For this review, take the finished solid that the model builds, in its own axes (mm). A direction names the side the tool comes from. Coordinates: 2 decimals unless noted, no trailing zeros. Loops run counter-clockwise (first coordinate to the right, second up) from the corner with the lowest first, then second, coordinate; pieces in that order, holes last. Notation, with made-up numbers: (-28, 61) -> (-23, 61) arc R28 cw to (-23, 80) -> close; hole circle Ø7 at (47.25, 51). An arc over 180 degrees is marked (long way). One line per item, written item: value.
from build123d import *

# Parameters (mm, degrees)
SKETCH2_R           = 1.5
BOSS_EXTRUDE1_DEPTH = 8.7
SKETCH3_R           = 4
SKETCH3_R_2         = 2.55
BOSS_EXTRUDE2_DEPTH = 2.5
BOSS_EXTRUDE3_START = -11.2
SKETCH3_3_R         = 4
SKETCH3_3_R_2       = 2.55
BOSS_EXTRUDE3_DEPTH = 2.5
CUT_EXTRUDE1_START  = -0.5
SKETCH2_3_R         = 5
SKETCH2_3_R_2       = 2.55
CUT_EXTRUDE1_DEPTH  = 9.7
BOSS_EXTRUDE4_START = -2.5
SKETCH2_4_R         = 2.55
BOSS_EXTRUDE4_DEPTH = 0.5
FILLET1_R           = 10
FILLET2_R           = 0.5
FILLET3_R           = 1


with BuildPart() as part:
    # Sketch2 → Boss-Extrude1 (new body)
    with BuildSketch(Plane(origin=(0, 0, 0), x_dir=(1, 0, 0), z_dir=(0, 1, 0))):
        with BuildLine():
            Line((3.9, 3.65), (-3.9, 3.65))
            Line((-3.9, 3.65), (-3.9, -3.65))
            Line((-3.9, -3.65), (-5, -3.65))
            Line((-5, -3.65), (-5, -6.15))
            Line((-5, -6.15), (-3.9, -6.15))
            Line((-3.9, -6.15), (-3.9, -21.871102431))
            ThreePointArc((-3.9, -21.871102431), (0, -20), (3.9, -21.871102431))
            Line((3.9, -21.871102431), (3.9, -6.15))
            Line((3.9, -6.15), (5, -6.15))
            Line((5, -6.15), (5, -3.65))
            Line((5, -3.65), (3.9, -3.65))
            Line((3.9, -3.65), (3.9, 3.65))
        make_face()
        with Locations(Location((0, 0.2, 0), (0, 0, 270))):
            Circle(SKETCH2_R, mode=Mode.SUBTRACT)
    extrude(amount=BOSS_EXTRUDE1_DEPTH)

    # Sketch3 → Boss-Extrude2 (add)
    # profile 1 of 4: a face of its own
    with BuildSketch(Plane(origin=(0, 8.7, 0), x_dir=(1, 0, 0), z_dir=(0, 1, 0))):
        Polygon((-5, -3.65), (-5, -6.15), (-3.9, -6.15), (3.9, -6.15), (5, -6.15), (5, -3.65), (3.9, -3.65), (-3.9, -3.65), align=None)
    # profile 2 of 4: a face of its own
    with BuildSketch(Plane(origin=(0, 8.7, 0), x_dir=(1, 0, 0), z_dir=(0, 1, 0))):
        with BuildLine():
            Line((3.9, -6.15), (-3.9, -6.15))
            Line((-3.9, -6.15), (-3.9, -21.871102431))
            ThreePointArc((-3.9, -21.871102431), (0, -20), (3.9, -21.871102431))
            Line((3.9, -21.871102431), (3.9, -6.15))
        make_face()
    # profile 3 of 4: a face of its own
    with BuildSketch(Plane(origin=(0, 8.7, 0), x_dir=(1, 0, 0), z_dir=(0, 1, 0))):
        with Locations((0, -25)):
            Circle(SKETCH3_R)
        with Locations(Location((0, -25, 0), (0, 0, 270))):
            Circle(SKETCH3_R_2, mode=Mode.SUBTRACT)
    # profile 4 of 4: a face of its own
    with BuildSketch(Plane(origin=(0, 8.7, 0), x_dir=(1, 0, 0), z_dir=(0, 1, 0))):
        with BuildLine():
            ThreePointArc((3.9, -21.871102431), (0, -20), (-3.9, -21.871102431))
            Line((-3.9, -21.871102431), (-3.9, -24.111180558))
            ThreePointArc((-3.9, -24.111180558), (0, -21), (3.9, -24.111180558))
            Line((3.9, -24.111180558), (3.9, -21.871102431))
        make_face()
    extrude(amount=BOSS_EXTRUDE2_DEPTH)

    # Sketch3<3> → Boss-Extrude3 (add)
    # profile 1 of 4: a face of its own
    with BuildSketch(Plane(origin=(0, 8.7, 0), x_dir=(1, 0, 0), z_dir=(0, 1, 0)).offset(BOSS_EXTRUDE3_START)):
        with Locations((0, -25)):
            Circle(SKETCH3_3_R)
        with Locations(Location((0, -25, 0), (0, 0, 270))):
            Circle(SKETCH3_3_R_2, mode=Mode.SUBTRACT)
    # profile 2 of 4: a face of its own
    with BuildSketch(Plane(origin=(0, 8.7, 0), x_dir=(1, 0, 0), z_dir=(0, 1, 0)).offset(BOSS_EXTRUDE3_START)):
        with BuildLine():
            ThreePointArc((3.9, -21.871102431), (0, -20), (-3.9, -21.871102431))
            Line((-3.9, -21.871102431), (-3.9, -24.111180558))
            ThreePointArc((-3.9, -24.111180558), (0, -21), (3.9, -24.111180558))
            Line((3.9, -24.111180558), (3.9, -21.871102431))
        make_face()
    # profile 3 of 4: a face of its own
    with BuildSketch(Plane(origin=(0, 8.7, 0), x_dir=(1, 0, 0), z_dir=(0, 1, 0)).offset(BOSS_EXTRUDE3_START)):
        with BuildLine():
            Line((3.9, -6.15), (-3.9, -6.15))
            Line((-3.9, -6.15), (-3.9, -21.871102431))
            ThreePointArc((-3.9, -21.871102431), (0, -20), (3.9, -21.871102431))
            Line((3.9, -21.871102431), (3.9, -6.15))
        make_face()
    # profile 4 of 4: a face of its own
    with BuildSketch(Plane(origin=(0, 8.7, 0), x_dir=(1, 0, 0), z_dir=(0, 1, 0)).offset(BOSS_EXTRUDE3_START)):
        Polygon((-5, -3.65), (-5, -6.15), (-3.9, -6.15), (3.9, -6.15), (5, -6.15), (5, -3.65), (3.9, -3.65), (-3.9, -3.65), align=None)
    extrude(amount=BOSS_EXTRUDE3_DEPTH)

    # Sketch2<3> → Cut-Extrude1 (cut)
    with BuildSketch(Plane(origin=(0, 0, 0), x_dir=(1, 0, 0), z_dir=(0, 1, 0)).offset(CUT_EXTRUDE1_START)):
        with Locations((0, -25)):
            Circle(SKETCH2_3_R)
        with Locations(Location((0, -25, 0), (0, 0, 270))):
            Circle(SKETCH2_3_R_2, mode=Mode.SUBTRACT)
    extrude(amount=CUT_EXTRUDE1_DEPTH, mode=Mode.SUBTRACT)

    # Sketch2<4> → Boss-Extrude4 (add)
    with BuildSketch(Plane(origin=(0, 0, 0), x_dir=(1, 0, 0), z_dir=(0, 1, 0)).offset(BOSS_EXTRUDE4_START)):
        with Locations(Location((0, -25, 0), (0, 0, 270))):
            Circle(SKETCH2_4_R)
    extrude(amount=BOSS_EXTRUDE4_DEPTH)

    # Fillet1
    # the kernel refuses this fillet: 10 mm, written as the material it adds along each edge
    with BuildSketch(Plane(origin=(-3.9, -2.5, 6.15), x_dir=(-1, 0, 0), z_dir=(0, 1, 0)), Plane(origin=(3.9, 11.2, 6.15), x_dir=(1, 0, 0), z_dir=(0, -1, 0))) as fillet1_piece_1:
        with BuildLine():
            CenterArc((10, 4.559605246), FILLET1_R, 180, 27.126753117)
            Line((0, 4.559605246), (-0.2, 4.559605246))
            Line((-0.2, 4.559605246), (-0.2, 0))
            Line((-0.2, 0), (0, -0.2))
            ThreePointArc((0, -0.2), (0.55, -0.2), (0.922, -0.091192105))
            Line((0.922, -0.091192105), (1.1, 0))
        make_face()
    extrude(amount=13.7)

    # Fillet2
    fillet2_edges = [part.edges().sort_by_distance(p)[0] for p in [
        (3.9, 4.35, 21.871102431),
        (-3.9, 4.35, 21.871102431),
    ]]
    fillet(fillet2_edges, radius=FILLET2_R)

    # Fillet3
    fillet3_edges = [part.edges().sort_by_distance(p)[0] for p in [
        (5, 4.35, 3.65),
        (-5, 4.35, 3.65),
        (-3.9, 4.35, -3.65),
        (3.9, 4.35, -3.65),
    ]]
    fillet(fillet3_edges, radius=FILLET3_R)


solid = part.part
1. Insertion check: pin 1 Ø6 at (y, z) = (7.5, 10.5) entering from +X; pin 2 Ø4 at (x, z) = (-0.5, 26) entering from +Y; pin 3 Ø5 at (y, z) = (6.5, 0.5) entering from +X; pin 4 Ø2 at (x, z) = (1.5, 0) entering from +Y. Each pin has a flat end and moves straight along its axis. Give the tip position at first contact, or say it passes through.
Return value:
pin 1: stops at x = 4.43
pin 2: stops at y = 11.2
pin 3: stops at x = 3.9
pin 4: stops at y = 8.7
2. Take a section at B-B, the plane x = 0. Give the boundary of the cut face in (y, z).
Return value:
outline: (-2.5, 3.65) -> (0, 3.65) -> (0, 1.3) -> (8.7, 1.3) -> (8.7, 3.65) -> (11.2, 3.65) -> (11.2, 22.45) -> (9.2, 22.45) -> (9.2, 20) -> (-0.5, 20) -> (-0.5, 22.45) -> (-2, 22.45) -> (-2, 27.55) -> (-0.5, 27.55) -> (-0.5, 29) -> (-2.5, 29) -> close; (0, -3.65) -> (8.7, -3.65) -> (8.7, -1.7) -> (0, -1.7) -> close; (9.2, 27.55) -> (11.2, 27.55) -> (11.2, 29) -> (9.2, 29) -> close
3. Take a section at D-D, the plane y = 2. Give the boundary of the cut face in (x, z).
Return value:
outline: (-5, 4.65) arc R1 ccw to (-4, 3.65) -> (-3.9, 3.65) -> (-3.9, -2.65) arc R1 ccw to (-2.9, -3.65) -> (2.9, -3.65) arc R1 ccw to (3.9, -2.65) -> (3.9, 3.65) -> (4, 3.65) arc R1 ccw to (5, 4.65) -> (5, 6.15) arc R10 cw to (3.9, 10.71) -> (3.9, 20.68) arc R0.5 ccw to (3.09, 21.07) arc R5 cw to (-3.09, 21.07) arc R0.5 ccw to (-3.9, 20.68) -> (-3.9, 10.71) arc R10 cw to (-5, 6.15) -> close; hole circle Ø3 at (0, -0.2)
4. Take a section at C-C, the plane z = -0.2. Give the boundary of the cut face in (x, y), and give its area (3 significant figures).
Return value:
outline: (-3.9, 0) -> (-1.5, 0) -> (-1.5, 8.7) -> (-3.9, 8.7) -> close; (1.5, 0) -> (3.9, 0) -> (3.9, 8.7) -> (1.5, 8.7) -> close
area: 41.8 mm2
5. For faces 4 (the cylindrical face through (3.61, 4.42, 21.13)), 5 (the flat face through (5, 4, 5)), 6 (the flat face through (-3.9, 4, 16)), 7 (the flat face through (0, -2, 25)), 8 (the flat face through (3.9, 4, 1)), list the 3-axis set-ups (+Z, -Z, +X, -X, +Y, -Y) from which the entire face can be reached by the end or side of a thin tool; tool diameter is ignored.
Return value:
face 4: +Z
face 5: +Z, -Z, +X, +Y, -Y
face 6: -X, +Y, -Y
face 7: +Y
face 8: -Z, +X, +Y, -Y
6. The part is to be moulded in two halves that separate along X. For faces 1 (the flat face through (0, 8.7, 2)), 2 (the cylindrical face through (0, 10, 29)), 3 (the cylindrical face through (0.112, 10.186, 22.452)), say which applies: pulls with the +X half, pulls with the -X half, needs draft (parallel to the pull), parting line crosses it, or undercut.
Return value:
face 1: needs draft
face 2: parting line crosses it
face 3: undercut
7. Take a section at A-A, the plane z = 25. Give the boundary of the cut face in (x, y).
Return value:
outline: (-4, -2.5) -> (4, -2.5) -> (4, -0.5) -> (2.55, -0.5) -> (2.55, -2) -> (-2.55, -2) -> (-2.55, -0.5) -> (-4, -0.5) -> close; (-4, 9.2) -> (-2.55, 9.2) -> (-2.55, 11.2) -> (-4, 11.2) -> close; (2.55, 9.2) -> (4, 9.2) -> (4, 11.2) -> (2.55, 11.2) -> close
8. To check wall thickness, follow probe 1 along X at (y, z) = (-0.95, 25); probe 2 along X at (y, z) = (5, -0.2); probe 3 along Z at (x, y) = (-0.5, -1). State the ranges of each line that lie inside material, in increasing order. Write a range as from..to.
Return value:
probe 1: x = -4..-2.55, 2.55..4
probe 2: x = -3.9..-1.5, 1.5..3.9
probe 3: z = 3.65..22.5, 27.5..28.97
